Check sheet for the modelled part. Datum: model origin and axes. Units: mm. A direction names the side the tool comes from. Give positions to 0.01 mm unless a question says otherwise; leave off trailing zeros. Write each loop counter-clockwise with the first axis right and the second up, starting at its lowest first coordinate (ties: lowest second). Pieces come first, ordered by that corner, then holes.
Autodesk Inventor part; units mm, degrees
ref_plane "YZ Plane" through (0, 0, 0) normal (1, 0, 0) x (0, 1, 0)
ref_plane "XZ Plane" through (0, 0, 0) normal (0, 1, 0) x (-1, 0, 0)
ref_plane "XY Plane" through (0, 0, 0) normal (0, 0, 1) x (1, 0, 0)
sketch "스케치1" plane through (0, 0, 0) normal (0, 0, 1) x (1, 0, 0)
  line L0 (80, -122.5) -> (0, -122.5)
  line L1 (80, 45) -> (110, 45)
  line L2 (110, 45) -> (110, -45)
  line L3 (110, -45) -> (80, -45)
  line L4 (80, 57.5) -> (80, 45)
  line L5 (80, -45) -> (80, -122.5)
  line L6 (40, 57.5) -> (40, -122.5)
  circle A0 centre (40, 47.0427) radius 7.5
  circle A1 centre (-7.0427, 0) radius 7.5
  circle A2 centre (40, -47.0427) radius 7.5
  circle A3 centre (87.0427, 0) radius 7.5
  circle A4 centre (40, 0) radius 7.5
  line L7 (0, 57.5) -> (80, 57.5)
  line L8 (0, 0) -> (0, 57.5)
  line L9 (0, 0) -> (0, -122.5)
  dimension "d0" = 80
  dimension "d3" = 45
  dimension "d4" = 45
  dimension "d13" = 360
  dimension "d14" = 0
  dimension "d15" = 47.0427
  dimension "d16" = 47.0427
  dimension "d21" = 15
  dimension "d31" = 122.5
  dimension "d36" = 12.5
  dimension "d37" = 30
extrude "돌출1" add sketch "스케치1" against normal blind 10 contours L0 L6 A2 A4 A0 L7 L4 L1 L2 L3 L5 | L0 L9 A1 L8 L7 L6 A0 A4 A2 | A2 L6 | L6 A2 | L9 L8 A1 | A4 L6 | L6 A4 | A0 L6 | L6 A0 | A3 picked at (0.0843, 1.4393)
extrude "돌출3" cut sketch "스케치1" against normal blind 40 contours A4 L6 | L6 A4
sketch "스케치2" plane through (0, -122.5, 0) normal (0, -1, 0) x (1, 0, 0)
  line L0 (0, 0) -> (80, 0)
  line L1 (15, 0) -> (15, 20)
  line L2 (15, 20) -> (65, 20)
  line L3 (65, 20) -> (65, 0)
  arc A0 (65, 20) -> (15, 20) centre (40, 20) ccw
  circle A1 centre (40, 20) radius 5
  point P0 (40, 0)
  dimension "d24" = 20
  dimension "d25" = 50
  dimension "d26" = 25
  dimension "d28" = 10
extrude "돌출4" add sketch "스케치2" against normal blind 10 contours L1 L2 A1 L3 L0 | A0 L2 A1
sketch "스케치3" plane through (0, 57.5, 0) normal (0, 1, 0) x (1, 0, 0)
  line L0 (15, 0) -> (15, -20)
  line L1 (65, -20) -> (65, 0)
  arc A0 (15, -20) -> (65, -20) centre (40, -20) ccw
  circle A1 centre (40, -20) radius 5
  line L2 (80, 0) -> (0, 0)
extrude "돌출5" add sketch "스케치3" against normal blind 10
properties part number "wheel_braket_front"
1) Scan lines: L1, parallel to X at y = -119.5, z = 20; L2, parallel to Z at x = 40, y = -115.25; L3, parallel to Y at x = 19.5, z = 22.5. Record each from-to range of solid material in increasing order.
2) Sectioned sample at C-C on z = -5. Record the boundary of the cut face in (x, y), then the cut area to 3 significant figures.
3) Draft check along X on faces 1 (the flat face through (80, -83, -5)), 2 (the flat face through (15, -118, 10)), 3 (the cylindrical face through (36, -118, 17)). Enter one of: +X half, -X half, draft (parallel to the pull), parting line (faces both ways), or undercut.
4) Access from +Z, -Z, +X, -X, +Y, -Y to the whole of each face (thin tool, end or side, straight path). Record for faces 4 (the flat face through (95, -45, -5)), 5 (the flat face through (80, 51, -5)), 6 (the flat face through (65, -118, 10)).
5) Gauge pin test, flat ends, axial feed: pin 1 (5 mm diameter, centred on x = 91, z = -5.5, fed in from +Y); pin 2 (8 mm diameter, centred on x = 85, y = 23, fed in from +Z); pin 3 (8 mm diameter, centred on y = -120, z = 13, fed in from -X); pin 4 (6 mm diameter, centred on x = 40, z = 20, fed in from -Y). Record the tip position at first contact, or that the pin passes through.
6) Sectioned sample at B-B on y = 0. Record the boundary of the cut face in (x, z), then the cut area to 3 significant figures.
7) Sectioned sample at A-A on x = 40. Record the boundary of the cut face in (y, z).
8) Sectioned sample at D-D on x = 101. Record the boundary of the cut face in (y, z), then the cut area to 3 significant figures.
Answers below:
1. L1: x = 15 to 35, 45 to 65
1. L2: z = -10 to 15, 25 to 45
1. L3: y = -122.5 to -112.5, 47.5 to 57.5
2. outline: (0, -122.5) - (80, -122.5) - (80, -45) - (110, -45) - (110, 45) - (80, 45) - (80, 57.5) - (0, 57.5) - close; hole circle Ø15 at (40, 0)
2. area: 16,900 mm2
3. face 1: +X half
3. face 2: -X half
3. face 3: undercut
4. face 4: +Z, -Z, +X, -Y
4. face 5: +Z, -Z, +X, +Y
4. face 6: +Z, +X, +Y, -Y
5. pin 1: stops at y = 45
5. pin 2: stops at z = 0
5. pin 3: stops at x = 15
5. pin 4: passes through
6. outline: (0, -10) - (32.5, -10) - (32.5, 0) - (0, 0) - close; (47.5, -10) - (110, -10) - (110, 0) - (47.5, 0) - close
6. area: 950 mm2
7. outline: (-122.5, -10) - (-7.5, -10) - (-7.5, 0) - (-112.5, 0) - (-112.5, 15) - (-122.5, 15) - close; (-122.5, 25) - (-112.5, 25) - (-112.5, 45) - (-122.5, 45) - close; (7.5, -10) - (57.5, -10) - (57.5, 15) - (47.5, 15) - (47.5, 0) - (7.5, 0) - close; (47.5, 25) - (57.5, 25) - (57.5, 45) - (47.5, 45) - close
8. outline: (-45, -10) - (45, -10) - (45, 0) - (-45, 0) - close
8. area: 900 mm2
